```python
from build123d import *

# Parameters (mm, degrees)
CROQUIS1_R              = 2.25
CROQUIS1_R_2            = 2
SALIENTE_EXTRUIR1_DEPTH = 3


with BuildPart() as part:
    # Croquis1 → Saliente-Extruir1 (new body)
    with BuildSketch(Plane.XY):
        Polygon((0, 0), (40, 0), (40, 110), (23, 110), (3, 110), (3, 93), (25, 93), (25, 17), (0, 17), align=None)
        with Locations((10, 8.5)):
            Circle(CROQUIS1_R, mode=Mode.SUBTRACT)
        with Locations((32.5, 32)):
            Circle(CROQUIS1_R_2, mode=Mode.SUBTRACT)
    extrude(amount=SALIENTE_EXTRUIR1_DEPTH)


solid = part.part
```
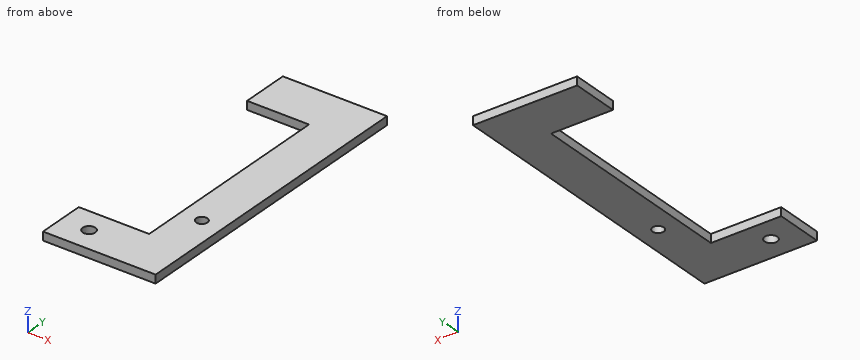
Verification items for the finished model (mm, model axes). Coordinates: 2 decimals unless noted, no trailing zeros. Write each loop counter-clockwise with the first axis right and the second up, starting at its lowest first coordinate (ties: lowest second). Pieces come first, ordered by that corner, then holes. Notation, with made-up numbers: (59, -11.75) - (109, -11.75) arc R27 ccw to (109, 23.25) - close; hole circle Ø11 at (3, 38). An arc over 180 degrees is marked (long way). One line per question, with ' | ' between items. Start each with the question number.
1. Material ranges on line 1 along Y through (x, z) = (10, 2.4); line 2 along Y through (x, z) = (5, 0.9); line 3 along Y through (x, z) = (32.5, 1.25), recorded low to high.
2. Section check D-D (y = 103). Enter the section's corners in (x, z).
3. Section check C-C (z = 1.85). Enter the section's corners in (x, y).
4. Section check B-B (x = 14). Enter the section's corners in (y, z).
5. Gauge pin test, flat ends, axial feed: P1, Ø2, axis at x = 31, y = 95, coming from the -Z side; P2, Ø1.5, axis at y = 20, z = 1.5, coming from the -X side; P3, Ø0.9, axis at y = 100, z = 2, coming from the -X side. Record the tip position at first contact, or that the pin passes through.
6. Section check A-A (y = 8.5). Enter the section's corners in (x, z), plus the area to 4 significant figures.
Computed values:
1) line 1: 0 to 6.25, 10.75 to 17, 93 to 110 | line 2: 0 to 17, 93 to 110 | line 3: 0 to 30, 34 to 110
2) outline: (3, 0) - (40, 0) - (40, 3) - (3, 3) - close
3) outline: (0, 0) - (40, 0) - (40, 110) - (3, 110) - (3, 93) - (25, 93) - (25, 17) - (0, 17) - close; hole circle Ø4.5 at (10, 8.5); hole circle Ø4 at (32.5, 32)
4) outline: (0, 0) - (17, 0) - (17, 3) - (0, 3) - close; (93, 0) - (110, 0) - (110, 3) - (93, 3) - close
5) P1: z = 0 | P2: x = 25 | P3: x = 3
6) outline: (0, 0) - (7.75, 0) - (7.75, 3) - (0, 3) - close; (12.25, 0) - (40, 0) - (40, 3) - (12.25, 3) - close | area: 106.5 mm²
